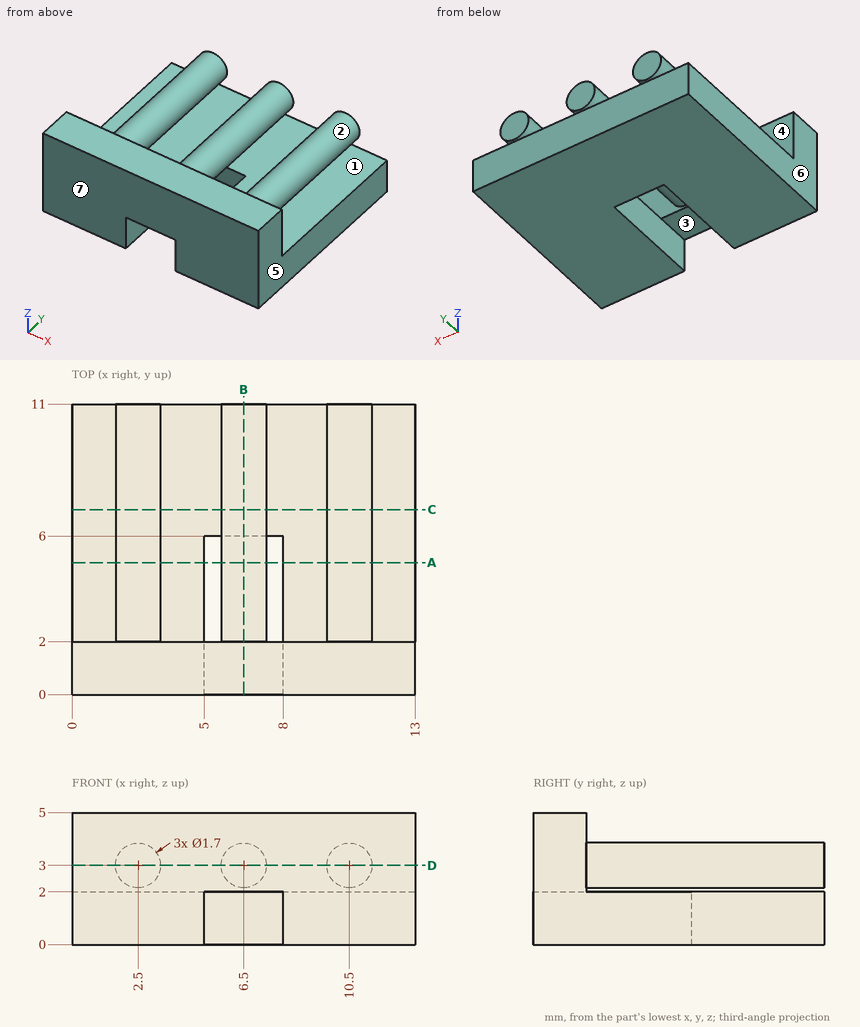
The figure shows three views and two pictorial views of one solid part (mm, origin at its lowest corner). Answer the questions. A direction names the side the tool comes from. Round coordinates to 2 decimals unless told otherwise and drop trailing zeros. Write each loop counter-clockwise with the first axis right and the second up, starting at its lowest first coordinate (ties: lowest second). Pieces come first, ordered by that corner, then holes. Notation, with made-up numbers: (14, 50) -> (57, 50) arc R19 ccw to (57, 61) -> close; hole circle Ø2 at (50.25, -24.5). An arc over 180 degrees is marked (long way). Answer as a JSON object with one key per item and string values. Group by question number.
Q1. Section A-A (y = 5) is taken. Write down the section's boundary in (x, z), plus the area to 3 significant figures.
Q2. Section B-B (x = 6.5) is taken. Write down the section's boundary in (y, z), plus the area to 3 significant figures.
Q3. Which of the six approach directions +Z, -Z, +X, -X, +Y, -Y give full straight-line access (tool end or side, diameter ignored) to the marked faces 1, 2 and 3?
Q4. Straight lines are drawn through the part: line 1 along X through (y, z) = (2.75, 0.2); line 2 along X through (y, z) = (6.25, 3.5); line 3 along X through (y, z) = (2.25, 2.25). For each, find the intervals that lie inside material, in ascending order.
Q5. Section D-D (z = 3) is taken. Write down the section's boundary in (x, y), plus the area to 3 significant figures.
Q6. Determine the mould class of the marked faces 4, 5, 6 and 7 for opening direction X: pulls with the +X half, pulls with the -X half, needs draft (parallel to the pull), parting line crosses it, or undercut.
Q7. Section C-C (y = 7) is taken. Write down the section's boundary in (x, z), plus the area to 3 significant figures.
Q8. Each of these flat-tipped pins is pushed along its axis until it touches: pin 1 Ø1 at (x, z) = (7, 0.5) entering from -Y; pin 2 Ø0.6 at (x, y) = (6, 0.5) entering from -Z; pin 3 Ø6 at (x, y) = (9.5, 7) entering from +Z. Where does it stop, or does it pass through?
Check values:
{
 "1": {"outline": "(0, 0) -> (5, 0) -> (5, 2) -> (0, 2) -> close; circle Ø1.7 at (2.5, 3); circle Ø1.7 at (6.5, 3); (8, 0) -> (13, 0) -> (13, 2) -> (8, 2) -> close; circle Ø1.7 at (10.5, 3)", "area": "26.8 mm^2"},
 "2": {"outline": "(0, 2) -> (2, 2) -> (2, 2.15) -> (11, 2.15) -> (11, 3.85) -> (2, 3.85) -> (2, 5) -> (0, 5) -> close; (6, 0) -> (11, 0) -> (11, 2) -> (6, 2) -> close", "area": "31.3 mm^2"},
 "3": {"face 1": "+X, -X, +Y", "face 2": "+Y", "face 3": "-Z, -Y"},
 "4": {"line 1": "0 to 5, 8 to 13", "line 2": "1.81 to 3.19, 5.81 to 7.19, 9.81 to 11.19", "line 3": "2.1 to 2.9, 6.1 to 6.9, 10.1 to 10.9"},
 "5": {"outline": "(0, 0) -> (13, 0) -> (13, 2) -> (11.35, 2) -> (11.35, 11) -> (9.65, 11) -> (9.65, 2) -> (7.35, 2) -> (7.35, 11) -> (5.65, 11) -> (5.65, 2) -> (3.35, 2) -> (3.35, 11) -> (1.65, 11) -> (1.65, 2) -> (0, 2) -> close", "area": "71.9 mm^2"},
 "6": {"face 4": "undercut", "face 5": "pulls with the +X half", "face 6": "pulls with the -X half", "face 7": "needs draft"},
 "7": {"outline": "(0, 0) -> (13, 0) -> (13, 2) -> (0, 2) -> close; circle Ø1.7 at (2.5, 3); circle Ø1.7 at (6.5, 3); circle Ø1.7 at (10.5, 3)", "area": "32.8 mm^2"},
 "8": {"pin 1": "y = 6", "pin 2": "z = 2", "pin 3": "z = 3.85"}
}
